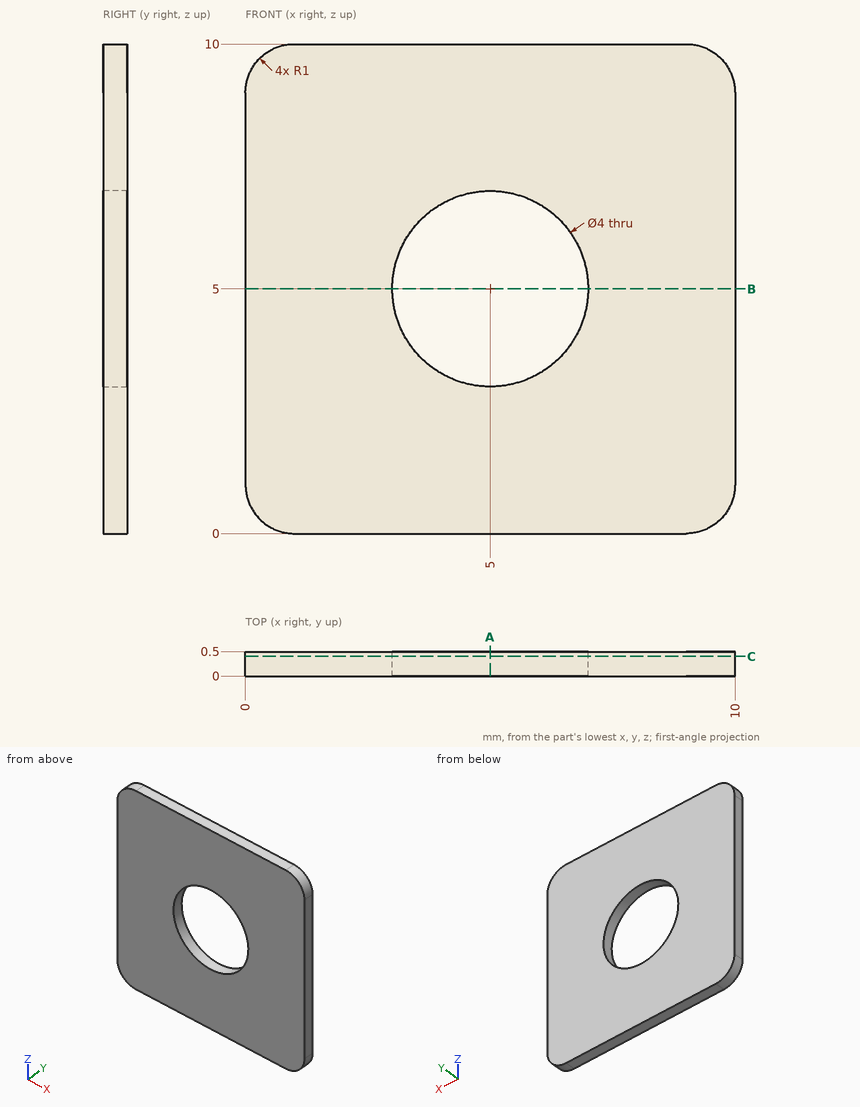
Here's the drawing with two shaded views (mm, measured from the low corner). I have some questions. Give positions to 0.01 mm unless a question says otherwise; leave off trailing zeros. Loops run counter-clockwise (first coordinate to the right, second up) from the corner with the lowest first, then second, coordinate; pieces in that order, holes last. Notation, with made-up numbers: M 80.25,24 L 129.25,24 A14 ccw 129.25,44 Z; hole C 79.25,30 d8. An arc over 180 degrees is marked long. Use one line per item in the form item = value. Start each with the question number.
Q1. If we section it at C-C (y = 0.4): Write out the boundary of the cut face in (x, z), then the cut area to 3 significant figures.
Q2. If we section it at A-A (x = 5): Write out the boundary of the cut face in (y, z), then the cut area to 3 significant figures.
Q3. If we section it at B-B (z = 5): Write out the boundary of the cut face in (x, y), then the cut area to 3 significant figures.
Q4. I need wall thicknesses on line 1 along X through (y, z) = (0.15, 5); line 2 along X through (y, z) = (0.35, 6.5). Which ranges of each line are inside material? Lowest first, please.
Taken from the geometry:
q1.outline = M 0,1 A1 ccw 1,0 L 9,0 A1 ccw 10,1 L 10,9 A1 ccw 9,10 L 1,10 A1 ccw 0,9 Z; hole C 5,5 d4
q1.area = 86.6 mm^2
q2.outline = M 0,0 L 0.5,0 L 0.5,3 L 0,3 Z; M 0,7 L 0.5,7 L 0.5,10 L 0,10 Z
q2.area = 3.00 mm^2
q3.outline = M 0,0 L 3,0 L 3,0.5 L 0,0.5 Z; M 7,0 L 10,0 L 10,0.5 L 7,0.5 Z
q3.area = 3.00 mm^2
q4.line_1 = 0 to 3, 7 to 10
q4.line_2 = 0 to 3.68, 6.32 to 10
